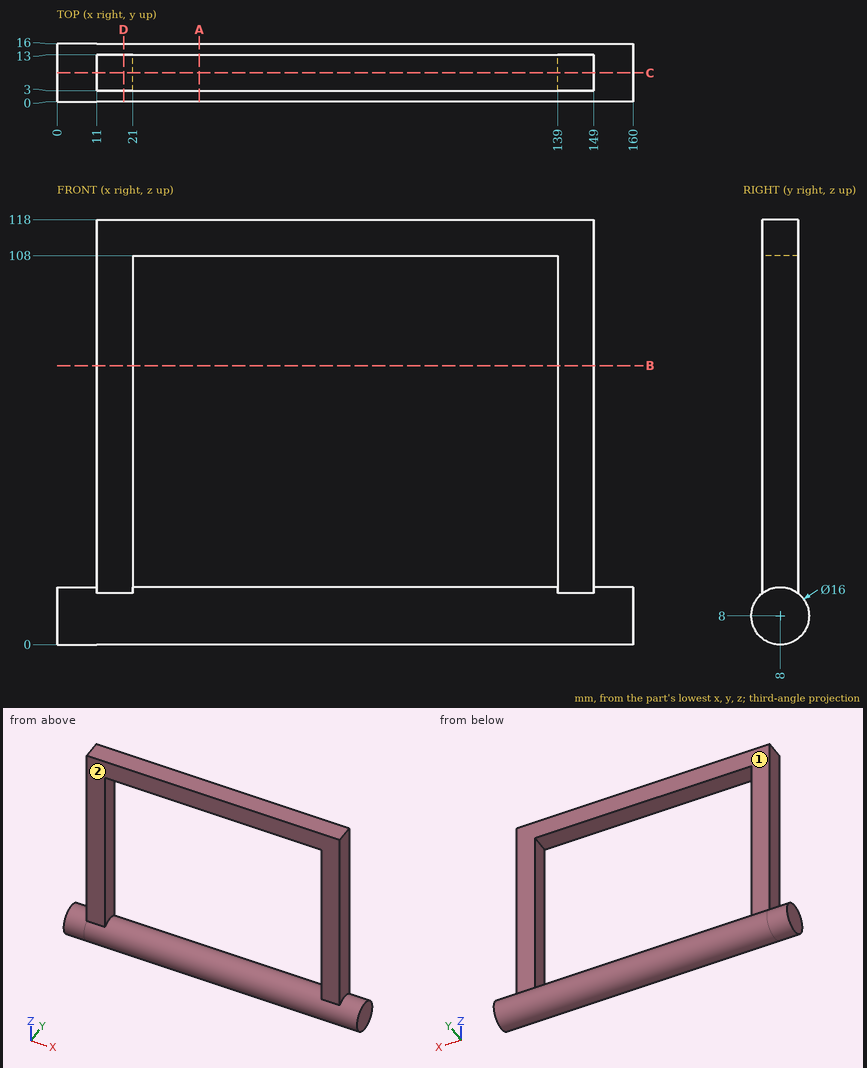
Source: three-view drawing plus pictorial views. Frame: mm from the lowest corner of the part. A direction names the side the tool comes from. Give positions to 0.01 mm unless a question says otherwise; leave off trailing zeros. Order: outer loops, then holes, each group sorted by start corner. A loop starts at its lowest first (then second) coordinate and runs counter-clockwise, first axis right, second up. Notation, with made-up numbers: (-35, 40) - (-11, 40) arc R11 ccw to (-11, 55) - close; hole circle Ø4 at (81, -38). An arc over 180 degrees is marked (long way). Answer as a JSON object with one key per item and string values. Group by question number.
Q1. Set-up query: the marked faces 1 and 2. Return all of +Z, -Z, +X, -X, +Y, -Y with unobstructed straight access to the full face (end or side cutting, diameter ignored); none if empty.
Q2. Line query: probe 1 along X at (y, z) = (6.75, 56); probe 2 along Z at (x, y) = (36.5, 11); probe 3 along Z at (x, y) = (140.5, 1.75). Output: solid intervals per line, ascending.
Q3. Cut plane C-C, the plane y = 8. Output: boundary loops of the cut face in (x, z).
Q4. Cut plane D-D, the plane x = 18.5. Output: boundary loops of the cut face in (y, z) (3 decimals), then the cut area to 3 significant figures.
Q5. Cut plane A-A, the plane x = 39.5. Output: boundary loops of the cut face in (y, z).
Q6. Cut plane B-B, the plane z = 77.5. Output: boundary loops of the cut face in (x, y).
Q7. First-contact query: pin 1 Ø6 at (x, y) = (72.5, 13) entering from -Z; pin 2 Ø3 at (y, z) = (10, 45.5) entering from +X; pin 3 Ø10 at (x, z) = (30, 65) entering from -Y; pin 4 Ø8 at (x, y) = (85.5, 5.5) entering from -Z. Flat tips, straight axial feed; report the tip coordinate or a pass-through.
Results:
{
 "1": {"face 1": "+Z, +X, -X, +Y", "face 2": "+Z, +X, -X, -Y"},
 "2": {"probe 1": "11 to 21, 139 to 149", "probe 2": "0.58 to 15.42, 108 to 118", "probe 3": "3.01 to 12.99"},
 "3": {"outline": "(0, 0) - (160, 0) - (160, 16) - (149, 16) - (149, 118) - (11, 118) - (11, 16) - (0, 16) - close; hole (21, 16) - (139, 16) - (139, 108) - (21, 108) - close"},
 "4": {"outline": "(3, 14.245) arc R8 ccw (long way) to (13, 14.245) - (13, 118) - (3, 118) - close", "area": "1,230 mm^2"},
 "5": {"outline": "circle Ø16 at (8, 8); (3, 108) - (13, 108) - (13, 118) - (3, 118) - close"},
 "6": {"outline": "(11, 3) - (21, 3) - (21, 13) - (11, 13) - close; (139, 3) - (149, 3) - (149, 13) - (139, 13) - close"},
 "7": {"pin 1": "z = 0.25", "pin 2": "x = 149", "pin 3": "through", "pin 4": "z = 0"}
}
